For this review, take the finished solid that the model builds, in its own axes (mm). Round coordinates to 2 decimals unless told otherwise and drop trailing zeros. Order: outer loops, then holes, each group sorted by start corner. A loop starts at its lowest first (then second) coordinate and runs counter-clockwise, first axis right, second up. Notation, with made-up numbers: M 10.25,25 L 49.25,25 A25 cw 49.25,58 Z; hole C -25,-26 d3. An arc over 180 degrees is marked long. Use a Markdown table: item, result.
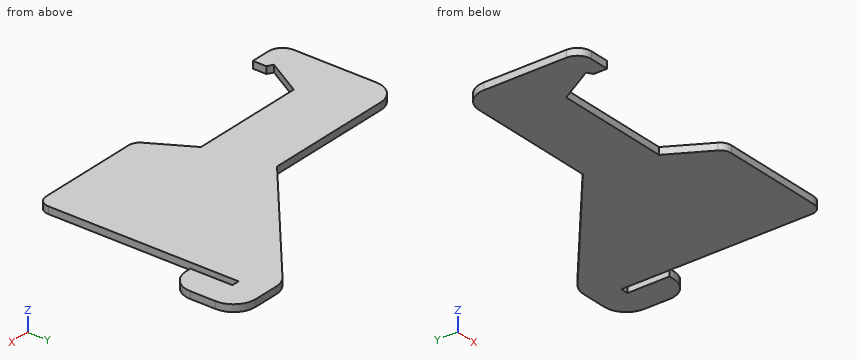
from build123d import *

# Parameters (mm, degrees)
BOSS_EXTRUDE1_DEPTH = 0.8001


with BuildPart() as part:
    # Sketch1 → Boss-Extrude1 (new body, symmetric)
    with BuildSketch(Plane.XY):
        with BuildLine():
            Line((27.250759249, 1.2954), (21.965453493, 10.449818102))
            Line((21.965453493, 10.449818102), (-4.418491784, 10.449818102))
            Line((-4.418491784, 10.449818102), (-9.22042678, 2.132622715))
            Line((-9.22042678, 2.132622715), (-7.95042678, 1.399387873))
            Line((-7.95042678, 1.399387873), (-7.95042678, -1.651))
            Line((-7.95042678, -1.651), (-12.39542678, -1.651))
            ThreePointArc((-12.39542678, -1.651), (-14.64049081, -0.72106403), (-15.57042678, 1.524))
            Line((-15.57042678, 1.524), (-15.57042678, 20.2692))
            ThreePointArc((-15.57042678, 20.2692), (-14.082529228, 23.861302448), (-10.49042678, 25.3492))
            Line((-10.49042678, 25.3492), (19.001320062, 25.3492))
            Line((19.001320062, 25.3492), (49.459807733, 50.906905771))
            ThreePointArc((49.459807733, 50.906905771), (50.987706462, 51.789038514), (52.72516879, 52.0954))
            Line((52.72516879, 52.0954), (58.4962, 52.0954))
            ThreePointArc((58.4962, 52.0954), (62.088302448, 50.607502448), (63.5762, 47.0154))
            Line((63.5762, 47.0154), (63.5762, 41.3004))
            ThreePointArc((63.5762, 41.3004), (62.088302448, 37.708297552), (58.4962, 36.2204))
            Line((58.4962, 36.2204), (57.2262, 36.2204))
            Line((57.2262, 36.2204), (57.2262, 45.7454))
            Line((57.2262, 45.7454), (55.4736, 45.7454))
            Line((55.4736, 45.7454), (55.4736, 2.5654))
            ThreePointArc((55.4736, 2.5654), (54.729651224, 0.769348776), (52.9336, 0.0254))
            Line((52.9336, 0.0254), (29.450463774, 0.0254))
            ThreePointArc((29.450463774, 0.0254), (28.180463774, 0.365695474), (27.250759249, 1.2954))
        make_face()
    extrude(amount=BOSS_EXTRUDE1_DEPTH, both=True)


solid = part.part
Q1. Add section A-A (y = 9.5). Write out the cut boundary in (x, z).
Determined:
| item | result |
|---|---|
| outline | M -15.57,-0.8 L -4.97,-0.8 L -4.97,0.8 L -15.57,0.8 Z; M 22.51,-0.8 L 55.47,-0.8 L 55.47,0.8 L 22.51,0.8 Z |
Q2. Wall thickness on line 1 along Y through (x, z) = (7, 0.25); line 2 along X through (y, z) = (17, -0.15); line 3 along Y through (x, z) = (58, -0.7): over which ranges is each line inside the solid? List them lowest first. Write a range as [from, to].
Determined:
| item | result |
|---|---|
| line 1 | y = [10.45, 25.35] |
| line 2 | x = [-15.57, 55.47] |
| line 3 | y = [36.22, 52.1] |
Q3. Add section C-C (y = 40.5). Write out the cut boundary in (x, z), then the cut area to 3 significant figures.
Determined:
| item | result |
|---|---|
| outline | M 37.06,-0.8 L 55.47,-0.8 L 55.47,0.8 L 37.06,0.8 Z; M 57.23,-0.8 L 63.51,-0.8 L 63.51,0.8 L 57.23,0.8 Z |
| area | 39.5 mm^2 |
Q4. Clearance check with flat-ended pins moving along their axes: pin 1 (0.5 mm diameter, centred on y = 17.5, z = -0.5, fed in from +X); pin 2 (0.8 mm diameter, centred on y = -0.5, z = 0, fed in from +X); pin 3 (0.8 mm diameter, centred on x = 44, z = 0, fed in from -Y). State where each tip first meets the part, or that it passes through.
Determined:
| item | result |
|---|---|
| pin 1 | stops at x = 55.47 |
| pin 2 | stops at x = -7.95 |
| pin 3 | stops at y = 0.03 |
Q5. Add section D-D (x = -3.5). Write out the cut boundary in (y, z), then the cut area to 3 significant figures.
Determined:
| item | result |
|---|---|
| outline | M 10.45,-0.8 L 25.35,-0.8 L 25.35,0.8 L 10.45,0.8 Z |
| area | 23.8 mm^2 |
